Verification items for this drawing (mm, ordinates from the low corner). Give positions to 0.01 mm unless a question says otherwise; leave off trailing zeros. Write each loop counter-clockwise with the first axis right and the second up, starting at its lowest first coordinate (ties: lowest second). Pieces come first, ordered by that corner, then holes. Notation, with made-up numbers: (49, 12) -> (86, 12) arc R15 cw to (86, 21) -> close; hole circle Ø4 at (49.5, 86.25). An arc over 180 degrees is marked (long way). Answer as a JSON object with one key per item and string values.
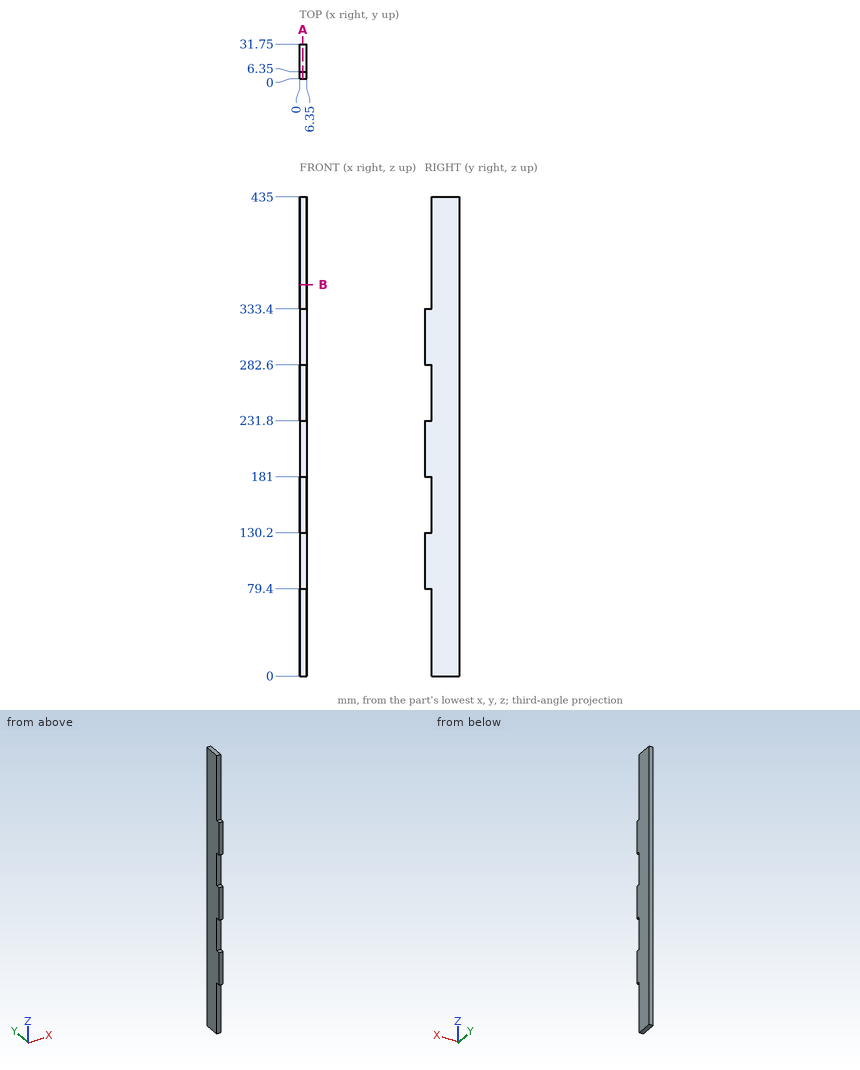
1. Go/stop test with flat-tipped pins: P1, Ø3, axis at x = 3, y = 4, coming from the -Z side; P2, Ø1.9, axis at x = 3, y = 4.5, coming from the +Z side; P3, Ø3, axis at x = 4, z = 36.5, coming from the -Y side. Record where each tip stops, or that it passes through.
Determined:
{"P1": "z = 79.4", "P2": "z = 333.4", "P3": "y = 6.35"}
2. Sectioned sample at A-A, the plane x = 3. Enter the section's corners in (y, z).
Determined:
{"outline": "(0, 79.4) -> (6.35, 79.4) -> (6.35, 0) -> (31.75, 0) -> (31.75, 435) -> (6.35, 435) -> (6.35, 333.4) -> (0, 333.4) -> (0, 282.6) -> (6.35, 282.6) -> (6.35, 231.8) -> (0, 231.8) -> (0, 181) -> (6.35, 181) -> (6.35, 130.2) -> (0, 130.2) -> close"}
3. Scan lines: L1, parallel to Z at x = 0.75, y = 5; L2, parallel to Y at x = 2, z = 164. Record each from-to range of solid material in increasing order. Write a range as [from, to].
Determined:
{"L1": "[79.4, 130.2], [181, 231.8], [282.6, 333.4]", "L2": "[6.35, 31.75]"}
4. Sectioned sample at B-B, the plane z = 355.5. Enter the section's corners in (x, y).
Determined:
{"outline": "(0, 6.35) -> (6.35, 6.35) -> (6.35, 31.75) -> (0, 31.75) -> close"}
